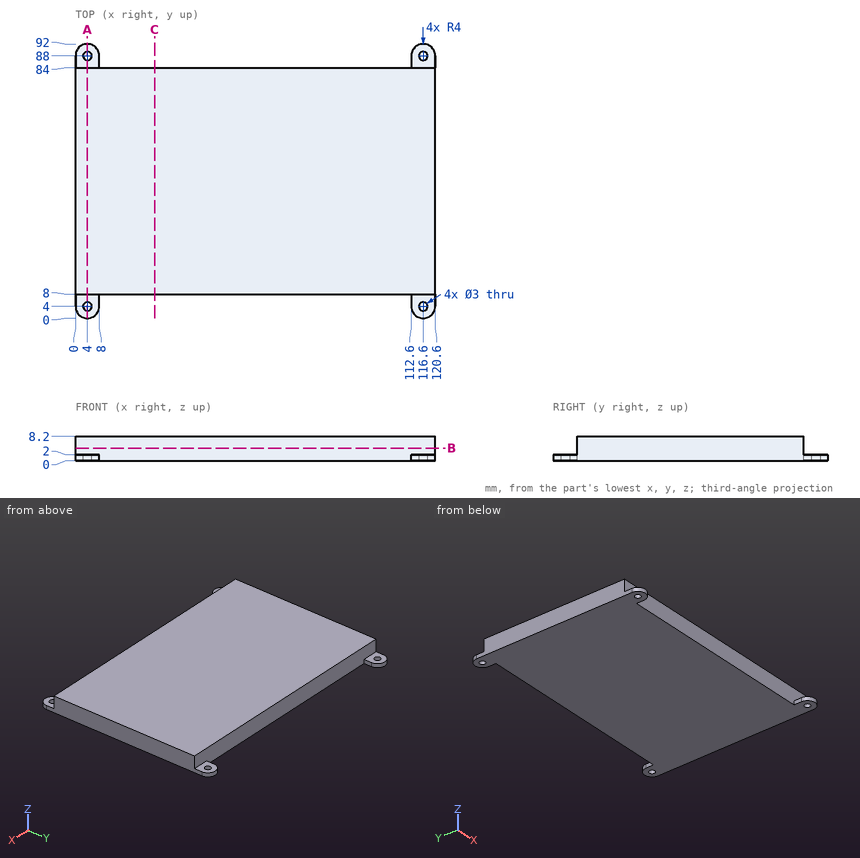
The drawing under review shows one solid part. Ordinate dimensions are in mm from its lowest x, y, z. Round coordinates to 2 decimals unless told otherwise and drop trailing zeros. Loops run counter-clockwise (first coordinate to the right, second up) from the corner with the lowest first, then second, coordinate; pieces in that order, holes last. Notation, with made-up numbers: (83, 88) - (130, 88) arc R21 cw to (130, 105) - close; hole circle Ø7 at (47, -33). An arc over 180 degrees is marked (long way). One line per question, with ' | ' between items.
Q1. For pin 1 (6.5 mm diameter, centred on x = 116, y = 4.5, fed in from +Z); pin 2 (6 mm diameter, centred on x = 27.5, y = 52, fed in from -Z); pin 3 (2 mm diameter, centred on x = 52.5, z = 3, fed in from -Y), all flat-tipped, find the tip position at first contact; note any pin that passes through.
Taken from the geometry:
pin 1: stops at z = 2 | pin 2: stops at z = 0 | pin 3: stops at y = 8
Q2. Take a section at C-C (x = 26.5). Give the boundary of the cut face in (y, z), and give its area (3 significant figures).
Taken from the geometry:
outline: (8, 0) - (84, 0) - (84, 8.2) - (8, 8.2) - close | area: 623 mm²
Q3. For line 1 along X through (y, z) = (88, 1); line 2 along Y through (x, z) = (4, 1.1); line 3 along Y through (x, z) = (73, 7), list the stretches that pass through material, from the lowest coordinate up. Write a range as [from, to].
Taken from the geometry:
line 1: x = [0, 2.5], [5.5, 8], [112.6, 115.1], [118.1, 120.6] | line 2: y = [0, 2.5], [5.5, 86.5], [89.5, 92] | line 3: y = [8, 84]
Q4. Take a section at A-A (x = 4). Give the boundary of the cut face in (y, z), and give its area (3 significant figures).
Taken from the geometry:
outline: (0, 0) - (2.5, 0) - (2.5, 2) - (0, 2) - close; (5.5, 0) - (86.5, 0) - (86.5, 2) - (84, 2) - (84, 8.2) - (8, 8.2) - (8, 2) - (5.5, 2) - close; (89.5, 0) - (92, 0) - (92, 2) - (89.5, 2) - close | area: 643 mm²
Q5. Take a section at B-B (z = 4.25). Give the boundary of the cut face in (x, y), and give its area (3 significant figures).
Taken from the geometry:
outline: (0, 8) - (120.6, 8) - (120.6, 84) - (0, 84) - close | area: 9,170 mm²
